from build123d import *

# Parameters (mm, degrees)
CUT_EXTRUDE1_DEPTH = 3.794
FILLET1_R          = 1.778


with BuildPart() as part:
    # Sketch2 → Revolve1 (revolve)
    with BuildSketch(Plane(origin=(0, 0, 0), x_dir=(1, 0, 0), z_dir=(0, 1, 0))):
        with BuildLine():
            Line((0.283958229, 14.224), (1.524, 13.949780367))
            ThreePointArc((1.524, 13.949780367), (0.382130108, 7.016390601), (0, 0))
            Line((0, 0), (-1.27, 0))
            ThreePointArc((-1.27, 0), (-0.880358119, 7.154316218), (0.283958229, 14.224))
        make_face()
    revolve(axis=Axis((0, 0, 0), (1, 0, 0)))

    # Sketch1 → Cut-Extrude1 (cut, through all)
    with BuildSketch(Plane(origin=(1.524, 0, 0), x_dir=(0, 0, -1), z_dir=(1, 0, 0))):
        with BuildLine():
            Line((-12.820693103, -6.160519812), (-5.457008659, -4.833450169))
            ThreePointArc((-5.457008659, -4.833450169), (-3.351086736, -6.473901585), (-0.795799518, -7.246232619))
            Line((-0.795799518, -7.246232619), (-1.174289533, -10.692611547))
            ThreePointArc((-1.174289533, -10.692611547), (5.59102597, -9.189740269), (10.03567463, -3.872484))
            Line((10.03567463, -3.872484), (6.8010357, -2.624328))
            ThreePointArc((6.8010357, -2.624328), (7.2898, 0), (6.8010357, 2.624328))
            Line((6.8010357, 2.624328), (10.03567463, 3.872484))
            ThreePointArc((10.03567463, 3.872484), (5.59102597, 9.189740269), (-1.174289533, 10.692611547))
            Line((-1.174289533, 10.692611547), (-0.795799518, 7.246232619))
            ThreePointArc((-0.795799518, 7.246232619), (-3.351086736, 6.473901585), (-5.457008659, 4.833450169))
            Line((-5.457008659, 4.833450169), (-12.820693103, 6.160519812))
            ThreePointArc((-12.820693103, 6.160519812), (-14.224, 0), (-12.820693103, -6.160519812))
        make_face()
    extrude(amount=-CUT_EXTRUDE1_DEPTH, mode=Mode.SUBTRACT)

    # Fillet1
    fillet1_edges = [part.edges().sort_by_distance(p)[0] for p in [
        (0.257994341, 10.692611547, 1.174289533),
        (0.257994341, 3.872484, -10.03567463),
        (0.257994341, -3.872484, -10.03567463),
        (0.257994341, -10.692611547, 1.174289533),
        (0.9039909, -6.135280444, 12.680644128),
        (0.9039909, 6.135280444, 12.680644128),
    ]]
    fillet(fillet1_edges, radius=FILLET1_R)


solid = part.part
Verification items for the finished model (mm, model axes). A direction names the side the tool comes from. Coordinates: 2 decimals unless noted, no trailing zeros. Order: outer loops, then holes, each group sorted by start corner. A loop starts at its lowest first (then second) coordinate and runs counter-clockwise, first axis right, second up. Notation, with made-up numbers: M 80,49 L 130,49 A9 cw 130,66 Z; hole C 67.5,70 d7. An arc over 180 degrees is marked long. One line per item, written item: value. Start each with the question number.
Item 1: Scan lines: probe 1 along Y at (x, z) = (0.55, 8.5); probe 2 along Y at (x, z) = (0.8, -2.5); probe 3 along X at (y, z) = (-7, -8.75). Record each from-to range of solid material in increasing order.
Item 2: Access from +Z, -Z, +X, -X, +Y, -Y to the whole of each face (thin tool, end or side, straight path). Record for faces 1 (the flat face through (0.1, 5.27, 7.87)), 2 (the cylindrical face through (-0.2, 6.5, 3.3)).
Item 3: Gauge pin test, flat ends, axial feed: pin 1 (1 mm diameter, centred on y = 0.5, z = -11, fed in from +X); pin 2 (12 mm diameter, centred on y = 1.5, z = 3, fed in from +X). Record the tip position at first contact, or that the pin passes through.
Item 4: Mould release check, pull along Z, two halves, no side actions. Record for faces 3 (the cylindrical face through (0.267, 9.154, -5.65)), 4 (the conical face through (1.326, -0.49, -13.985)), 5 (the cylindrical face through (0.1, -10.2, 0.45)), 6 (the flat face through (-0.121, 2.893, -7.496)): released by +Z, released by -Z, zero draft, split by the parting line, or undercut.
Item 5: Sectioned sample at B-B (y = 0). Enter the section's corners in (x, z).
Item 6: Sectioned sample at A-A (z = 0). Enter the section's corners in (x, y), then the cut area to 3 significant figures.
Conclusion:
1. probe 1: y = -11.33 to -5.38, 5.38 to 11.33
1. probe 2: y = -13.89 to -10.46, 10.46 to 13.89
1. probe 3: x = -0.31 to 0.98
2. face 1: +Z, +X, -X
2. face 2: +X, -X
3. pin 1: stops at x = 1.03
3. pin 2: stops at x = 0.67
4. face 3: undercut
4. face 4: split by the parting line
4. face 5: undercut
4. face 6: released by +Z
5. outline: M -0.87,-7.29 A65.88 ccw 0.28,-14.22 L 1.52,-13.95 A64.61 cw 0.41,-7.29 Z
6. outline: M -0.42,-10.53 A65.88 ccw 0.28,-14.22 L 1.52,-13.95 A64.61 cw 0.86,-10.53 Z; M -0.42,10.53 L 0.86,10.53 A64.61 cw 1.52,13.95 L 0.28,14.22 A65.88 ccw Z
6. area: 9.21 mm^2
